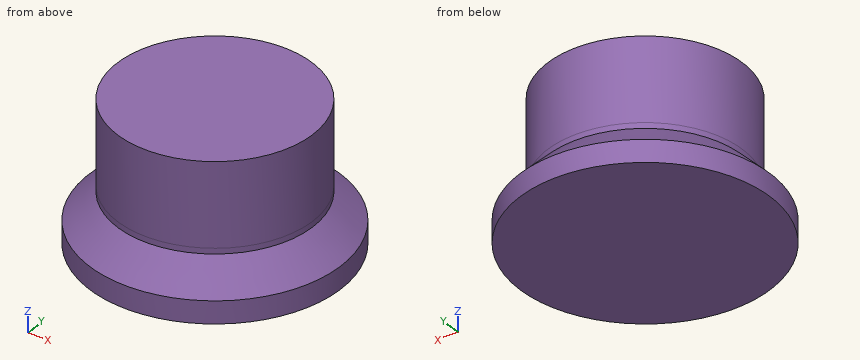
from build123d import *

# Parameters (mm, degrees)
F0_R        = 22.5
F0_R_2      = 17.5
F1_DEPTH    = 10
F2_DEPTH    = 25
F3_S5_R     = 17.5
F3_T6_DEPTH = 33


# Not quite as in the source:
# - a fillet or chamfer that OpenCascade refuses, or shapes differently, is made with other operations: its cross-section is extruded or revolved along the edge and cut away or added


with BuildPart() as f1:
    # F0 (on Top) → F1 (new body)
    with BuildSketch(Plane.XY):
        Circle(F0_R)
        Circle(F0_R_2, mode=Mode.SUBTRACT)
    extrude(amount=F1_DEPTH)

    # F0 (on Top) → F2 (join)
    with BuildSketch(Plane.XY):
        Circle(F0_R_2)
    extrude(amount=F2_DEPTH)

    # F3: chamfer of 6 on 1 edges, made by hand


with BuildPart() as f3_tool2:
    # F3_s3 → F3_t4 (revolve)
    with BuildSketch(Plane.XZ):
        Polygon((22.5, 4), (16.5, 10), (22.5, 10), align=None)
    revolve(axis=Axis((0, 0, 10), (0, 0, 1)))

    # F3_s5 → F3_t6 (cut, symmetric)
    with BuildSketch(Plane.XY.offset(7)):
        Circle(F3_S5_R)
    extrude(amount=F3_T6_DEPTH, both=True, mode=Mode.SUBTRACT)


with BuildPart() as f1_1:
    add(f1.part)

    # F3_t1: cut F3_tool2
    add(f3_tool2.part, mode=Mode.SUBTRACT)


solid = f1_1.part
The model under review builds one solid part; all positions refer to its coordinate system, in mm. Give positions to 0.01 mm unless a question says otherwise; leave off trailing zeros. Loops run counter-clockwise (first coordinate to the right, second up) from the corner with the lowest first, then second, coordinate; pieces in that order, holes last. Notation, with made-up numbers: (83, 45.25) -> (113, 45.25) arc R29 cw to (113, 81.25) -> close; hole circle Ø7 at (12, 76.5). An arc over 180 degrees is marked (long way). Answer as a JSON object with one key per item and string values. Group by question number.
Q1. Take a section at C-C (z = 16.25). Write out the cut boundary in (x, y), plus the area to 3 significant figures.
Q2. Insertion check: pin 1 (8 mm diameter, centred on y = 14, z = 10.5, fed in from -X); pin 2 (2 mm diameter, centred on y = 2, z = 7, fed in from +X); pin 3 (1 mm diameter, centred on x = 12.5, y = -18, fed in from -Z); pin 4 (3 mm diameter, centred on y = -7, z = 9, fed in from -X). Each pin has a flat end and moves straight along its axis. Give the tip position at first contact, or say it passes through.
Q3. Wall thickness on line 1 along X through (y, z) = (-9, 6); line 2 along Z through (x, y) = (-17.5, 14); line 3 along X through (y, z) = (-6.5, 13.75): over which ranges is each line inside the solid? List them lowest first.
Q4. Take a section at A-A (x = 0). Write out the cut boundary in (y, z).
Answer below:
{
 "1": {"outline": "circle Ø35 at (0, 0)", "area": "962 mm2"},
 "2": {"pin 1": "stops at x = -15.33", "pin 2": "stops at x = 20.41", "pin 3": "stops at z = 0", "pin 4": "stops at x = -17.76"},
 "3": {"line 1": "x = -18.42 to 18.42", "line 2": "z = 0 to 4.09", "line 3": "x = -16.25 to 16.25"},
 "4": {"outline": "(-22.5, 0) -> (22.5, 0) -> (22.5, 4) -> (17.5, 9) -> (17.5, 25) -> (-17.5, 25) -> (-17.5, 9) -> (-22.5, 4) -> close"}
}
